Could you check a few things on this model? Use its own coordinates, in mm. Face numbers are marked on the shaded views. Round coordinates to 2 decimals unless told otherwise and drop trailing zeros. Write each loop counter-clockwise with the first axis right and the second up, starting at its lowest first coordinate (ties: lowest second). Pieces come first, ordered by that corner, then holes. Notation, with made-up numbers: M 55,64 L 78,64 A10 ccw 78,76 Z; hole C 66.25,3.5 d4. An arc over 180 degrees is marked long. One line per item, written item: value. Start each with the question number.
(1) I want a section at D-D on y = 1.3. Please give me the cut outline in (x, z).
(2) I'm going to push flat-ended pins straight in: pin 1 Ø3.5 at (x, z) = (-1, -22.5) entering from +Y; pin 2 Ø1.5 at (x, y) = (-2.5, 2) entering from -Z; pin 3 Ø3.5 at (x, z) = (-1, -29) entering from +Y. Where does each tip first touch, or does it pass through?
(3) If I drill on L1, parallel to Y at x = 2.5, z = -28.5; L2, parallel to Z at x = 1.25, y = 4.4; L3, parallel to Y at x = 0.5, z = -22, over which ranges is the centre line in solid material (lowest first)?
(4) Thinking about a two-plate mould opening in Z: for the marked faces 1 and 2, which applies, released by +Z, released by -Z, zero draft, split by the parting line, or undercut?
(5) I want a section at C-C on x = -1.5. Please give me the cut outline in (y, z).
(6) I want a section at B-B on z = -17.5. Please give me the cut outline in (x, y).
(7) I want a section at A-A on y = 4.45. Please give me the cut outline in (x, z).
```python
from build123d import *

# Parameters (mm, degrees)
EXTRUDE_1_DEPTH     = 6
CUT_EXTRUDE_1_DEPTH = 2.1
SKETCH_4_R          = 3.5
CUT_EXTRUDE_2_DEPTH = 2.1


with BuildPart() as part:
    # Эскиз2 → Бобышка-Вытянуть1 (new body)
    with BuildSketch(Plane(origin=(0, 0, 0), x_dir=(1, 0, 0), z_dir=(0, 1, 0))):
        with BuildLine():
            Line((-5.696343687, 30.010357476), (-5.499915116, -19.989642524))
            ThreePointArc((-5.499915116, -19.989642524), (0.021649418, -25.467993105), (5.5, -19.946428571))
            Line((5.5, -19.946428571), (5.303571429, 30.053571429))
            ThreePointArc((5.303571429, 30.053571429), (-0.217993105, 35.53192201), (-5.696343687, 30.010357476))
        make_face()
    extrude(amount=EXTRUDE_1_DEPTH)

    # Эскиз3 → Вырез-Вытянуть1 (cut)
    with BuildSketch(Plane(origin=(0, 6, 0), x_dir=(1, 0, 0), z_dir=(0, 1, 0))):
        with BuildLine():
            Line((-3.680431468, 29.698156009), (-2.122840442, 13.441174328))
            ThreePointArc((-2.122840442, 13.441174328), (-0.124100309, 11.631937444), (1.860362916, 13.456822627))
            Line((1.860362916, 13.456822627), (3.290174408, 29.725540532))
            ThreePointArc((3.290174408, 29.725540532), (-0.210136023, 33.531937444), (-3.680431468, 29.698156009))
        make_face()
    extrude(amount=-CUT_EXTRUDE_1_DEPTH, mode=Mode.SUBTRACT)

    # Эскиз4 → Вырез-Вытянуть2 (cut)
    with BuildSketch(Plane(origin=(0, 3.9, 0), x_dir=(1, 0, 0), z_dir=(0, 1, 0))):
        with Locations(Location((-0.196386129, 30.031964452, 0), (0, 0, 270))):
            Circle(SKETCH_4_R)
    extrude(amount=-CUT_EXTRUDE_2_DEPTH, mode=Mode.SUBTRACT)


solid = part.part
```
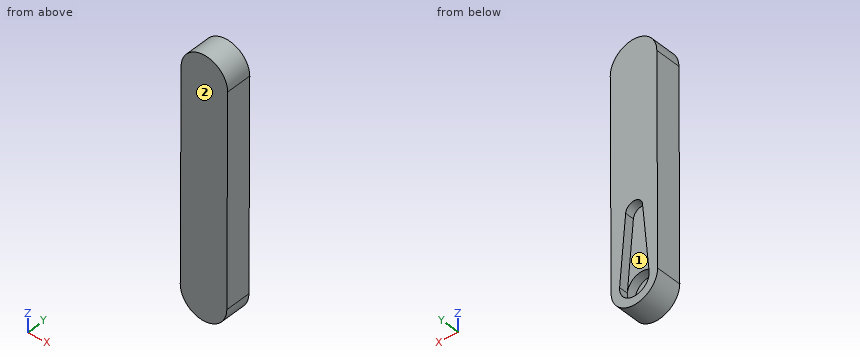
Found:
1. outline: M -5.7,-30.01 A5.5 ccw 5.3,-30.05 L 5.5,19.95 A5.5 ccw -5.5,19.99 Z
2. pin 1: stops at y = 3.9
2. pin 2: stops at z = -35.31
2. pin 3: stops at y = 1.8
3. L1: y = 0 to 1.8
3. L2: z = -35.34 to -33.22, -12.19 to 25.32
3. L3: y = 0 to 3.9
4. face 1: undercut
4. face 2: zero draft
5. outline: M 0,-35.38 L 6,-35.38 L 6,-33.28 L 1.8,-33.28 L 1.8,-26.78 L 3.9,-26.78 L 3.9,-12.17 L 6,-12.17 L 6,25.26 L 0,25.26 Z
6. outline: M -5.65,0 L 5.35,0 L 5.35,6 L 2.22,6 L 2.22,3.9 L -2.51,3.9 L -2.51,6 L -5.65,6 Z
7. outline: M -5.7,-30.01 A5.5 ccw 5.3,-30.05 L 5.5,19.95 A5.5 ccw -5.5,19.99 Z; hole M -3.68,-29.7 A3.5 ccw long 3.29,-29.73 L 1.86,-13.46 A2 ccw -2.12,-13.44 Z
